Geometry: final body of the model. Coordinates: model frame, mm. A direction names the side the tool comes from. Round coordinates to 2 decimals unless told otherwise and drop trailing zeros. Order: outer loops, then holes, each group sorted by start corner. A loop starts at its lowest first (then second) coordinate and runs counter-clockwise, first axis right, second up. Notation, with made-up numbers: M 19.5,-8 L 58.5,-8 A16 cw 58.5,23 Z; hole C 73.5,33 d7. An arc over 180 degrees is marked long. Return JSON: item names as keys, results as strings. Group by question number.
Q1. Access query for faces 1 (the face through (10, -1, 1)), 2 (the face through (-3, -6.83, -1)), 3 (the face through (4, 0, 0)). Directions: +Z, -Z, +X, -X, +Y, -Y. A direction counts if a zero-diameter tool reaches every point of the face in a straight line with its end or side. Return the directions, or none.
Q2. Ray query, probe 1 along X at (y, z) = (-0.75, 2.5); probe 2 along X at (y, z) = (-2.25, 0.5); probe 3 along Y at (x, z) = (6.5, -2.5). Return the intervals inside material, ascending.
Q3. Contact query for flat-ended pins moving along their axis: pin 1 (1 mm diameter, centred on x = 5, z = -1, fed in from -Y); pin 2 (3 mm diameter, centred on x = 8, z = 1, fed in from +Y). Output: stop coordinate, or through.
Q4. Cut plane C-C on z = -1.75. Output: boundary loops of the cut face in (x, y).
Q5. Cut plane A-A on y = -7. Output: boundary loops of the cut face in (x, z) (3 decimals), and give its area (3 significant figures).
Q6. Cut plane D-D on y = -2.75. Output: boundary loops of the cut face in (x, z) (3 decimals), and give its area (3 significant figures).
Q7. Cut plane B-B on x = 0.5. Output: boundary loops of the cut face in (y, z) (3 decimals).
Q8. Mould query, pull axis X, two halves, no side actions, for faces 4 (the face through (10, -6.83, 1)), 5 (the face through (4, -4, -3.665)). Classes: released by +X, released by -X, zero draft, split by the parting line, or undercut.
```python
from build123d import *

# Parameters (mm, degrees)
F0_R     = 2.45
F1_DEPTH = 7.83
F2_DEPTH = 1
F3_R     = 3.1
F3_R_2   = 2.45
F4_DEPTH = 1


with BuildPart() as f1:
    # F0 (on Front) → F1 (new body)
    with BuildSketch(Plane.XZ):
        with BuildLine():
            ThreePointArc((-4.1537828283, 0), (-3.0803291813, -2.591546353), (-0.4887828283, -3.665))
            Line((-0.4887828283, -3.665), (7.8475505051, -3.665))
            ThreePointArc((7.8475505051, -3.665), (10.4390968581, -2.591546353), (11.5125505051, 0))
            ThreePointArc((11.5125505051, 0), (10.4390968581, 2.591546353), (7.8475505051, 3.665))
            Line((7.8475505051, 3.665), (3.6792171717, 3.665))
            Line((3.6792171717, 3.665), (-0.4887828283, 3.665))
            ThreePointArc((-0.4887828283, 3.665), (-3.0803291813, 2.591546353), (-4.1537828283, 0))
        make_face()
        with BuildLine():
            ThreePointArc((-1.8208784206, -2.665), (-3.3372828283, 0), (-1.8208784206, 2.665))
            ThreePointArc((-1.8208784206, 2.665), (-0.2372828283, 3.1), (1.346312764, 2.665))
            ThreePointArc((1.346312764, 2.665), (2.8627171717, 0), (1.346312764, -2.665))
            ThreePointArc((1.346312764, -2.665), (-0.2372828283, -3.1), (-1.8208784206, -2.665))
        make_face(mode=Mode.SUBTRACT)
        with BuildLine():
            ThreePointArc((6.0122882461, -2.665), (4.4958838384, 0), (6.0122882461, 2.665))
            ThreePointArc((6.0122882461, 2.665), (10.6958838384, 0), (6.0122882461, -2.665))
        make_face(mode=Mode.SUBTRACT)
        with BuildLine():
            ThreePointArc((1.346312764, 2.665), (-0.2372828283, 3.1), (-1.8208784206, 2.665))
            ThreePointArc((-1.8208784206, 2.665), (-3.3372828283, 0), (-1.8208784206, -2.665))
            ThreePointArc((-1.8208784206, -2.665), (-0.2372828283, -3.1), (1.346312764, -2.665))
            ThreePointArc((1.346312764, -2.665), (2.8627171717, 0), (1.346312764, 2.665))
        make_face()
        with Locations((-0.2372828283, 0)):
            Circle(F0_R, mode=Mode.SUBTRACT)
        with BuildLine():
            ThreePointArc((6.0122882461, -2.665), (10.6958838384, 0), (6.0122882461, 2.665))
            ThreePointArc((6.0122882461, 2.665), (4.4958838384, 0), (6.0122882461, -2.665))
        make_face()
        with Locations((7.5958838384, 0)):
            Circle(F0_R, mode=Mode.SUBTRACT)
    extrude(amount=F1_DEPTH)

    # F0 (on Front) → F2 (cut)
    with BuildSketch(Plane.XZ):
        with BuildLine():
            ThreePointArc((1.346312764, 2.665), (-0.2372828283, 3.1), (-1.8208784206, 2.665))
            ThreePointArc((-1.8208784206, 2.665), (-3.3372828283, 0), (-1.8208784206, -2.665))
            ThreePointArc((-1.8208784206, -2.665), (-0.2372828283, -3.1), (1.346312764, -2.665))
            ThreePointArc((1.346312764, -2.665), (2.8627171717, 0), (1.346312764, 2.665))
        make_face()
        with Locations((-0.2372828283, 0)):
            Circle(F0_R, mode=Mode.SUBTRACT)
        with BuildLine():
            ThreePointArc((6.0122882461, -2.665), (10.6958838384, 0), (6.0122882461, 2.665))
            ThreePointArc((6.0122882461, 2.665), (4.4958838384, 0), (6.0122882461, -2.665))
        make_face()
        with Locations((7.5958838384, 0)):
            Circle(F0_R, mode=Mode.SUBTRACT)
    extrude(amount=F2_DEPTH, mode=Mode.SUBTRACT)

    # F3 (on face) → F4 (cut)
    with BuildSketch(Plane.XZ.offset(7.83)):
        with Locations((-0.2372828283, 0)):
            Circle(F3_R)
        with Locations((-0.2372828283, 0)):
            Circle(F3_R_2, mode=Mode.SUBTRACT)
        with Locations((7.5958838384, 0)):
            Circle(F3_R)
        with Locations((7.5958838384, 0)):
            Circle(F3_R_2, mode=Mode.SUBTRACT)
    extrude(amount=-F4_DEPTH, mode=Mode.SUBTRACT)


solid = f1.part
```
Result sheet:
{
 "1": {"face 1": "+Y", "face 2": "-Y", "face 3": "+Z, -Z, +X, -X, +Y"},
 "2": {"probe 1": "x = -3.17 to -2.07, 1.6 to 5.76, 9.43 to 10.53", "probe 2": "x = -4.12 to -2.64, 2.16 to 5.2, 9.99 to 11.48", "probe 3": "y = -6.83 to -1"},
 "3": {"pin 1": "stops at y = -7.83", "pin 2": "stops at y = -1"},
 "4": {"outline": "M -3.71,-7.83 L -2.8,-7.83 L -2.8,-6.83 L -1.95,-6.83 L -1.95,-1 L -2.8,-1 L -2.8,0 L -3.71,0 Z; M 1.48,-6.83 L 2.32,-6.83 L 2.32,-7.83 L 5.04,-7.83 L 5.04,-6.83 L 5.88,-6.83 L 5.88,-1 L 5.04,-1 L 5.04,0 L 2.32,0 L 2.32,-1 L 1.48,-1 Z; M 9.31,-6.83 L 10.15,-6.83 L 10.15,-7.83 L 11.07,-7.83 L 11.07,0 L 10.15,0 L 10.15,-1 L 9.31,-1 Z"},
 "5": {"outline": "M -0.489,-3.665 L 7.848,-3.665 A3.665 ccw 7.848,3.665 L -0.489,3.665 A3.665 ccw Z; hole C -0.237,0 d6.2; hole C 7.596,0 d6.2", "area": "42.9 mm²"},
 "6": {"outline": "M -0.489,-3.665 L 7.848,-3.665 A3.665 ccw 7.848,3.665 L -0.489,3.665 A3.665 ccw Z; hole C -0.237,0 d4.9; hole C 7.596,0 d4.9", "area": "65.6 mm²"},
 "7": {"outline": "M -7.83,-3.665 L 0,-3.665 L 0,-3.011 L -1,-3.011 L -1,-2.336 L -6.83,-2.336 L -6.83,-3.011 L -7.83,-3.011 Z; M -7.83,3.011 L -6.83,3.011 L -6.83,2.336 L -1,2.336 L -1,3.011 L 0,3.011 L 0,3.665 L -7.83,3.665 Z"},
 "8": {"face 4": "undercut", "face 5": "zero draft"}
}
